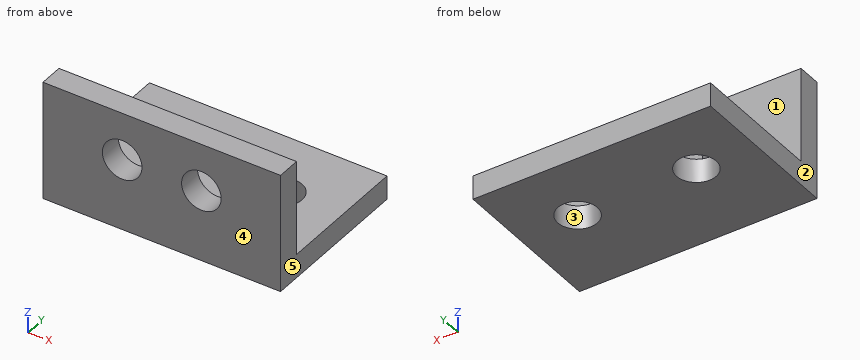
from build123d import *

# Parameters (mm, degrees)
BOSS_EXTRUDE1_DEPTH = 38.1
SKETCH3_R           = 3.175
CUT_EXTRUDE1_DEPTH  = 49.26
SKETCH4_R           = 3.175
CUT_EXTRUDE2_DEPTH  = 25.4


with BuildPart() as part:
    # Sketch2 → Boss-Extrude1 (new body)
    with BuildSketch(Plane(origin=(0, 0, 0), x_dir=(0, 0, -1), z_dir=(1, 0, 0))):
        Polygon((0, 0), (-19.05, 0), (-19.05, 3.81), (-3.81, 3.81), (-3.81, 25.4), (0, 25.4), align=None)
    extrude(amount=BOSS_EXTRUDE1_DEPTH)

    # Sketch3 → Cut-Extrude1 (cut, through all)
    with BuildSketch(Plane.XY.offset(3.81)):
        with Locations((9.525, 14.605)):
            Circle(SKETCH3_R)
        with Locations(Location((28.575, 14.605, 0), (0, 0, 180))):
            Circle(SKETCH3_R)
    extrude(amount=-CUT_EXTRUDE1_DEPTH, mode=Mode.SUBTRACT)

    # Sketch4 → Cut-Extrude2 (cut)
    with BuildSketch(Plane(origin=(0, 0, 0), x_dir=(-1, 0, 0), z_dir=(0, -1, 0))):
        with Locations(Location((-12.7, -11.43, 0), (0, 0, 90))):
            Circle(SKETCH4_R)
        with Locations(Location((-25.4, -11.43, 0), (0, 0, 90))):
            Circle(SKETCH4_R)
    extrude(amount=-CUT_EXTRUDE2_DEPTH, mode=Mode.SUBTRACT)


solid = part.part
The model under review builds one solid part; all positions refer to its coordinate system, in mm. Face numbers are marked on the shaded views. A direction names the side the tool comes from. Round coordinates to 2 decimals unless told otherwise and drop trailing zeros. Loops run counter-clockwise (first coordinate to the right, second up) from the corner with the lowest first, then second, coordinate; pieces in that order, holes last. Notation, with made-up numbers: (-28.75, -36) -> (-20.75, -36) arc R36 ccw to (-20.75, 0) -> close; hole circle Ø3 at (51.5, -6.75). An arc over 180 degrees is marked (long way). Write item = value, one per line. Start each with the question number.
Item 1: Insertion check: pin 1 (1 mm diameter, centred on x = 27, y = 5, fed in from -Z); pin 2 (5 mm diameter, centred on x = 26, y = 20, fed in from +Z); pin 3 (5 mm diameter, centred on x = 28.575, y = 14.605, fed in from +Z) (3 decimals). Each pin has a flat end and moves straight along its axis. Give the tip position at first contact, or say it passes through.
Item 2: To check wall thickness, follow L1, parallel to X at y = 2.1, z = 11.43 (3 decimals); L2, parallel to X at y = 13.5, z = 1.75; L3, parallel to Z at x = 22, y = 22. State the ranges of each line that lie inside material, in increasing order.
Item 3: Take a section at D-D on x = 20. Give the boundary of the cut face in (y, z).
Item 4: For the marked faces 1 and 2, list the 3-axis set-ups (+Z, -Z, +X, -X, +Y, -Y) from which the entire face can be reached by the end or side of a thin tool; tool diameter is ignored.
Item 5: Mouldability with a two-part tool opening along X and no side actions: class the marked faces 3, 4 and 5 as released by +X, released by -X, zero draft, split by the parting line, or undercut.
Item 6: Take a section at C-C on y = 15.5. Give the boundary of the cut face in (x, z).
Item 7: Take a section at B-B on x = 14.5. Give the boundary of the cut face in (y, z), plus the area to 3 significant figures.
Item 8: Take a section at A-A on z = 11.43. Give the boundary of the cut face in (x, y) (3 decimals), plus the area to 3 significant figures.
Result:
q1.pin_1 = 0
q1.pin_2 = 3.81
q1.pin_3 = through
q2.L1 = 0 to 9.525, 15.875 to 22.225, 28.575 to 38.1
q2.L2 = 0 to 6.55, 12.5 to 25.6, 31.55 to 38.1
q2.L3 = 0 to 3.81
q3.outline = (0, 0) -> (25.4, 0) -> (25.4, 3.81) -> (3.81, 3.81) -> (3.81, 19.05) -> (0, 19.05) -> close
q4.face_1 = +Z, +X, -X, +Y
q4.face_2 = +Z, -Z, -X, +Y, -Y
q5.face_3 = undercut
q5.face_4 = zero draft
q5.face_5 = released by +X
q6.outline = (0, 0) -> (6.48, 0) -> (6.48, 3.81) -> (0, 3.81) -> close; (12.57, 0) -> (25.53, 0) -> (25.53, 3.81) -> (12.57, 3.81) -> close; (31.62, 0) -> (38.1, 0) -> (38.1, 3.81) -> (31.62, 3.81) -> close
q7.outline = (0, 0) -> (25.4, 0) -> (25.4, 3.81) -> (3.81, 3.81) -> (3.81, 8.81) -> (0, 8.81) -> close; (0, 14.05) -> (3.81, 14.05) -> (3.81, 19.05) -> (0, 19.05) -> close
q7.area = 135 mm²
q8.outline = (0, 0) -> (9.525, 0) -> (9.525, 3.81) -> (0, 3.81) -> close; (15.875, 0) -> (22.225, 0) -> (22.225, 3.81) -> (15.875, 3.81) -> close; (28.575, 0) -> (38.1, 0) -> (38.1, 3.81) -> (28.575, 3.81) -> close
q8.area = 96.8 mm²
